from build123d import *

# Parameters (mm, degrees)
CUT_EXTRUDE_1_REACH = 29
SKETCH_2_R          = 4.15


with BuildPart() as part:
    # 스케치1 → 회전1 (revolve)
    with BuildSketch(Plane(origin=(0, 0, 0), x_dir=(0, 0, -1), z_dir=(1, 0, 0)), mode=Mode.PRIVATE) as revolve_1_sk:
        with BuildLine():
            Line((1, 13.5), (85, 13.5))
            Line((85, 13.5), (90.996839672, 12.279929179))
            ThreePointArc((90.996839672, 12.279929179), (93.87196322, 10.543832299), (95, 7.380305656))
            Line((95, 7.380305656), (95, 0))
            Line((95, 0), (0, 0))
            Line((0, 0), (0, 12.5))
            Line((0, 12.5), (1, 13.5))
        make_face()
    revolve(revolve_1_sk.sketch.rotate(Axis((0, 0, 0), (0, 0, -1)), 90), axis=Axis((0, 0, 0), (0, 0, -1)))  # turned: the seam where the file's is

    # 스케치2 → 컷-돌출1 (cut, up to next)
    with BuildSketch(Plane(origin=(0, 13.5, 0), x_dir=(1, 0, 0), z_dir=(0, 1, 0)), mode=Mode.PRIVATE) as cut_extrude_1_sk1:
        with Locations(Location((0, 10, 0), (0, 0, 270))):  # turned: the seam where the file's is
            Circle(SKETCH_2_R)
    cut_extrude_1_tool1 = extrude(cut_extrude_1_sk1.sketch, amount=-CUT_EXTRUDE_1_REACH, mode=Mode.PRIVATE) & part.part
    add(cut_extrude_1_tool1.solids().sort_by_distance((0, 13.5, -10))[0], mode=Mode.SUBTRACT)


solid = part.part
CAD build for the part. Positions are in the model's coordinates, mm. Round coordinates to 2 decimals unless told otherwise and drop trailing zeros. Order: outer loops, then holes, each group sorted by start corner. A loop starts at its lowest first (then second) coordinate and runs counter-clockwise, first axis right, second up. Notation, with made-up numbers: (2.25, 3.25) - (31.25, 3.25) arc R31 ccw to (31.25, 39.25) - close; hole circle Ø9 at (60, -25). An arc over 180 degrees is marked (long way). Return JSON: item names as keys, results as strings.
(1) Wall check: probe 1 along Z at (x, y) = (0, 2.25); probe 2 along X at (y, z) = (-6.25, -10); probe 3 along X at (y, z) = (0.5, -10). Give the ranges that are in metal, low to high. Write a range as from..to.
Answer key:
{"probe 1": "z = -95..-14.15, -5.85..0", "probe 2": "x = -11.97..-4.15, 4.15..11.97", "probe 3": "x = -13.49..-4.15, 4.15..13.49"}
(2) Cut at A-A (x = 0). Give the cut face in (y, z).
Answer key:
{"outline": "(-13.5, -85) - (-12.28, -91) arc R5 ccw to (-7.38, -95) - (7.38, -95) arc R5 ccw to (12.28, -91) - (13.5, -85) - (13.5, -14.15) - (-13.5, -14.15) - close; (-13.5, -5.85) - (13.5, -5.85) - (13.5, -1) - (12.5, 0) - (-12.5, 0) - (-13.5, -1) - close"}
(3) Pin check, flat tips, straight feed: pin 1 Ø3 at (x, z) = (7, -51.5) entering from +Y; pin 2 Ø5 at (x, y) = (8, 9.5) entering from +Z; pin 3 Ø2 at (x, z) = (-8, -47.5) entering from -Y; pin 4 Ø6 at (y, z) = (4.5, -76) entering from -X. Stop position of each tip, or through.
Answer key:
{"pin 1": "stops at y = 12.33", "pin 2": "stops at z = 0", "pin 3": "stops at y = -11.54", "pin 4": "stops at x = -13.42"}
(4) Pull direction Z, two halves, no side cores. Call faces 1 (the face through (0, 0, 0)), 2 (the face through (0, 0, -95)), 3 (the face through (-2.53, 0.19, -13.29)): +Z half, -Z half, draft (parallel to the pull), parting line (faces both ways), or undercut.
Answer key:
{"face 1": "+Z half", "face 2": "-Z half", "face 3": "undercut"}
(5) Cut at C-C (z = -10). Give the cut face in (x, y), then the cut area to 3 significant figures.
Answer key:
{"outline": "(-4.15, -12.85) - (-4.15, 12.85) arc R13.5 ccw to start; (4.15, -12.85) arc R13.5 ccw to (4.15, 12.85) - close", "area": "352 mm^2"}
(6) Cut at D-D (z = -27.5). Give the cut face in (x, y).
Answer key:
{"outline": "circle Ø27 at (0, 0)"}
(7) Cut at B-B (y = 0). Give the cut face in (x, z).
Answer key:
{"outline": "(-13.5, -85) - (-12.28, -91) arc R5 ccw to (-7.38, -95) - (7.38, -95) arc R5 ccw to (12.28, -91) - (13.5, -85) - (13.5, -1) - (12.5, 0) - (-12.5, 0) - (-13.5, -1) - close; hole circle Ø8.3 at (0, -10)"}
